Verification items for this drawing (mm, ordinates from the low corner). A direction names the side the tool comes from. Give positions to 0.01 mm unless a question says otherwise; leave off trailing zeros. Write each loop counter-clockwise with the first axis right and the second up, starting at its lowest first coordinate (ties: lowest second). Pieces come first, ordered by that corner, then holes. Notation, with made-up numbers: (23.5, -26) -> (73.5, -26) arc R11 ccw to (73.5, -13) -> close; hole circle Ø4 at (-6, 52.5). An arc over 180 degrees is marked (long way). Answer as a JSON object with one key per item and string values.
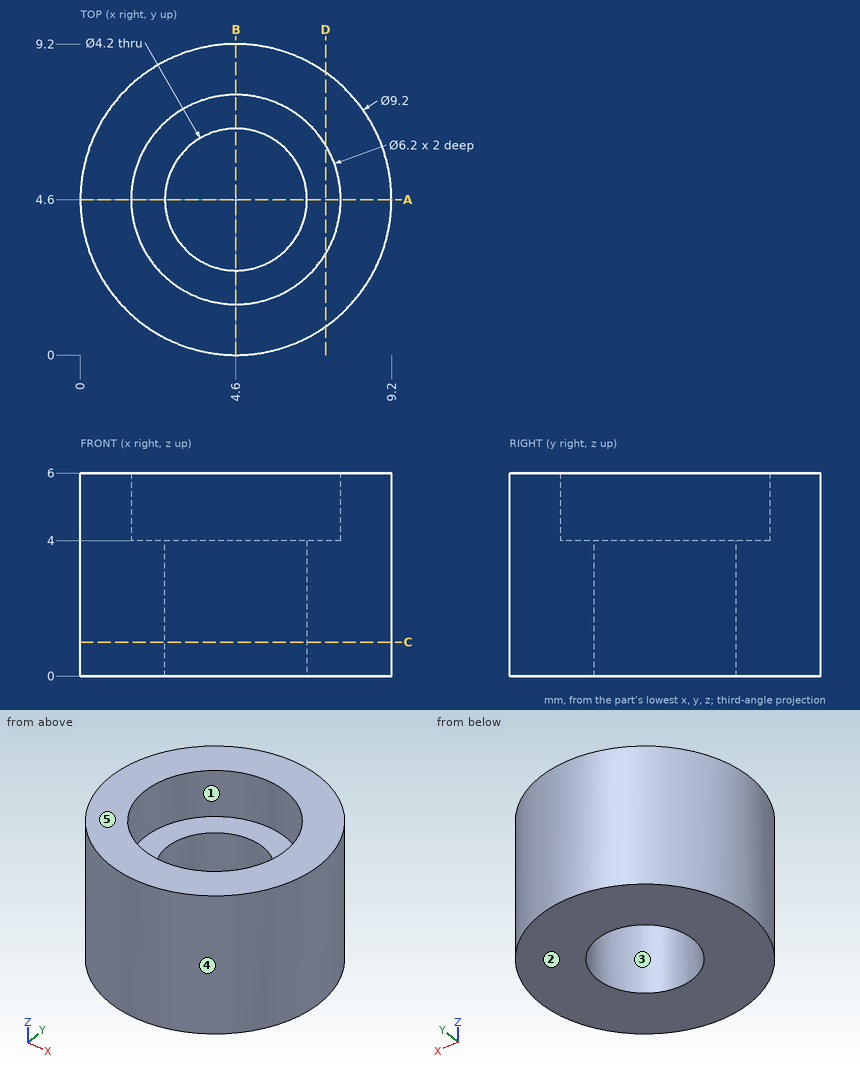
1. Access from +Z, -Z, +X, -X, +Y, -Y to the whole of each face (thin tool, end or side, straight path). Record for the marked faces 1 and 2.
Determined:
{"face 1": "+Z", "face 2": "-Z, +X, -X, +Y, -Y"}
2. Go/stop test with a flat-tipped pin: P1, Ø3, axis at x = 4.5, y = 3.5, coming from the +Z side. Record where the tip stops, or that it passes through.
Determined:
{"P1": "z = 4"}
3. Sectioned sample at C-C, the plane z = 1. Enter the section's corners in (x, y), plus the area to 3 significant figures.
Determined:
{"outline": "circle Ø9.2 at (4.6, 4.6); hole circle Ø4.2 at (4.6, 4.6)", "area": "52.6 mm^2"}
4. Scan lines: L1, parallel to Y at x = 4.6, z = 4.5; L2, parallel to Y at x = 4.6, z = 1.9. Record each from-to range of solid material in increasing order. Write a range as [from, to].
Determined:
{"L1": "[0, 1.5], [7.7, 9.2]", "L2": "[0, 2.5], [6.7, 9.2]"}
5. Sectioned sample at A-A, the plane y = 4.6. Enter the section's corners in (x, z).
Determined:
{"outline": "(0, 0) -> (2.5, 0) -> (2.5, 4) -> (1.5, 4) -> (1.5, 6) -> (0, 6) -> close; (6.7, 0) -> (9.2, 0) -> (9.2, 6) -> (7.7, 6) -> (7.7, 4) -> (6.7, 4) -> close"}
6. Mould release check, pull along Y, two halves, no side actions. Record for the marked faces 3, 4 and 5: released by +Y, released by -Y, zero draft, split by the parting line, or undercut.
Determined:
{"face 3": "undercut", "face 4": "split by the parting line", "face 5": "zero draft"}
7. Sectioned sample at D-D, the plane x = 7.25. Enter the section's corners in (y, z).
Determined:
{"outline": "(0.84, 0) -> (8.36, 0) -> (8.36, 6) -> (6.21, 6) -> (6.21, 4) -> (2.99, 4) -> (2.99, 6) -> (0.84, 6) -> close"}
